Autodesk Inventor part; units mm, degrees
ref_plane "YZ Plane" through (0, 0, 0) normal (1, 0, 0) x (0, 1, 0)
ref_plane "XZ Plane" through (0, 0, 0) normal (0, 1, 0) x (-1, 0, 0)
ref_plane "XY Plane" through (0, 0, 0) normal (0, 0, 1) x (1, 0, 0)
sketch "Sketch1" plane through (0, 0, 0) normal (0, 1, 0) x (-1, 0, 0)
  line L0 (0, 0) -> (-20, 0)
  line L1 (-20, 0) -> (-20, -10)
  line L2 (-20, -10) -> (0, -10)
  line L3 (0, -10) -> (0, 0)
  line L4 (-15, -3) -> (-5, -3) construction
  line L5 (-15, -4) -> (-5, -4)
  line L6 (-5, -2) -> (-15, -2)
  arc A0 (-15, -2) -> (-15, -4) centre (-15, -3) ccw
  arc A1 (-5, -4) -> (-5, -2) centre (-5, -3) ccw
  point P0 (-10, -3)
  point P1 (-10, -10)
  point P2 (-20, -5)
  dimension "d0" = 20
  dimension "d1" = 10
  dimension "d2" = 2
  dimension "d3" = 10
  dimension "d10" = 2
extrude "Extrusion1" add sketch "Sketch1" along normal blind 3
sketch "Sketch2" plane through (20, 0, -10) normal (0, 0, -1) x (-1, 0, 0)
  line L0 (0, 0) -> (0, 3)
  line L1 (0, 0) -> (-20, 0)
  line L2 (-20, 0) -> (-20, 10)
  line L3 (-20, 10) -> (0, 10)
  line L4 (0, 10) -> (0, 0)
  point P0 (20, 0)
  point P1 (0, 3)
  dimension "d6" = 10
  dimension "d7" = 20
extrude "Extrusion2" add sketch "Sketch2" against normal blind 3
fillet "Fillet1" radius 1 5 edges at (0, 1.5, -10) (0, 1.5, 0) (20, 1.5, 0) (20, 3, -8.5) (20, 1.5, -7)
fillet "Fillet2" radius 1 2 edges at (19.5, 3, -7) (20.5, 3, -7)
fillet "Fillet3" radius 1 3 edges at (20, 10, -8.5) (40, 10, -8.5) (40, 0, -8.5)
properties part number "servo attachment"
Here's how the part is built. I have some questions about the finished solid (model axes, mm). A direction names the side the tool comes from. Round coordinates to 2 decimals unless told otherwise and drop trailing zeros. Order: outer loops, then holes, each group sorted by start corner. A loop starts at its lowest first (then second) coordinate and runs counter-clockwise, first axis right, second up. Notation, with made-up numbers: M 61.5,-6 L 116.5,-6 A9 ccw 116.5,11 Z; hole C 35,-36 d4. An arc over 180 degrees is marked long. Answer in a Markdown table with one row per item.
Item 1: For faces 5 (the face through (4, 1, -3)), 6 (the face through (20, 7, -9)), 7 (the face through (15, 0, -6)), which set-ups out of +Z, -Z, +X, -X, +Y, -Y let a thin tool reach every point of the face, with its end or its side?
A:
| item | result |
|---|---|
| face 5 | +Y, -Y |
| face 6 | +Z, -Z, -X, +Y |
| face 7 | +Z, -Z, +X, -X, -Y |
Item 2: Imagine slicing it at A-A, the plane x = 11.5. Write out the boundary of the cut face in (y, z).
A:
| item | result |
|---|---|
| outline | M 0,-10 L 3,-10 L 3,-4 L 0,-4 Z; M 0,-2 L 3,-2 L 3,0 L 0,0 Z |
Item 3: Thinking about a two-plate mould opening in X: for faces 1 (the face through (10, 1, -2)), 2 (the face through (25, 4, -10)), 3 (the face through (16, 1, -3)), 4 (the face through (20.301, 9.715, -8.479)), which applies, +X half, -X half, draft (parallel to the pull), parting line (faces both ways), or undercut?
A:
| item | result |
|---|---|
| face 1 | undercut |
| face 2 | draft |
| face 3 | undercut |
| face 4 | -X half |
Item 4: Imagine slicing it at D-D, the plane x = 35.5. Write out the boundary of the cut face in (y, z).
A:
| item | result |
|---|---|
| outline | M 0,-10 L 10,-10 L 10,-7 L 0,-7 Z |
Item 5: Imagine slicing it at B-B, the plane z = -3. Write out the boundary of the cut face in (x, y), and give its area (3 significant figures).
A:
| item | result |
|---|---|
| outline | M 0,0 L 4,0 L 4,3 L 0,3 Z; M 16,0 L 20,0 L 20,3 L 16,3 Z |
| area | 24.0 mm2 |
Item 6: If I drill on L1, parallel to Y at x = 3, z = -5.5; L2, parallel to X at y = 4.5, z = -9; L3, parallel to X at y = 1.5, z = -5.75, over which ranges is the centre line in solid material (lowest first)? Write a range as from..to.
A:
| item | result |
|---|---|
| L1 | y = 0..3 |
| L2 | x = 20..40 |
| L3 | x = 0..20 |
Item 7: I'm going to push flat-ended pins straight in: pin 1 (1.5 mm diameter, centred on y = 7, z = -8, fed in from -X); pin 2 (2 mm diameter, centred on y = 6, z = -5.5, fed in from -X); pin 3 (6 mm diameter, centred on y = 4, z = -1.5, fed in from +X); pin 4 (3 mm diameter, centred on x = 10, z = -4, fed in from +Y). Where does each tip first touch, or does it pass through?
A:
| item | result |
|---|---|
| pin 1 | stops at x = 20 |
| pin 2 | passes through |
| pin 3 | stops at x = 20 |
| pin 4 | stops at y = 3 |
Item 8: Imagine slicing it at C-C, the plane y = 4.5. Write out the boundary of the cut face in (x, z).
A:
| item | result |
|---|---|
| outline | M 20,-10 L 40,-10 L 40,-7 L 20,-7 Z |
